Could you check a few things on this model? Use its own coordinates, in mm. Give positions to 0.01 mm unless a question says otherwise; leave off trailing zeros. Order: outer loops, then holes, each group sorted by start corner. A loop starts at its lowest first (then second) coordinate and runs counter-clockwise, first axis right, second up.
from build123d import *

# Parameters (mm, degrees)
SKETCH1_W           = 3
SKETCH1_H           = 6
SKETCH1_W_2         = 6
SKETCH1_H_2         = 3
SKETCH1_W_3         = 50
SKETCH1_H_3         = 50
BOSS_EXTRUDE1_DEPTH = 3
SKETCH2_R           = 2
SKETCH2_W           = 20
SKETCH2_H           = 6.4
CUT_EXTRUDE1_DEPTH  = 76.013332148


with BuildPart() as part:
    # Sketch1 → Boss-Extrude1 (new body)
    with BuildSketch(Plane(origin=(0, 0, 0), x_dir=(1, 0, 0), z_dir=(0, 1, 0))):
        with Locations((-51.5, 9)):
            Rectangle(SKETCH1_W, SKETCH1_H)
        with Locations((-51.5, 25)):
            Rectangle(SKETCH1_W, SKETCH1_H)
        with Locations((-51.5, 41)):
            Rectangle(SKETCH1_W, SKETCH1_H)
        with Locations((-41, 51.5)):
            Rectangle(SKETCH1_W_2, SKETCH1_H_2)
        with Locations((-25, 25)):
            Rectangle(SKETCH1_W_3, SKETCH1_H_3)
        with Locations((-25, 51.5)):
            Rectangle(SKETCH1_W_2, SKETCH1_H_2)
        with Locations((-9, 51.5)):
            Rectangle(SKETCH1_W_2, SKETCH1_H_2)
        with Locations((1.5, 41)):
            Rectangle(SKETCH1_W, SKETCH1_H)
        with Locations((1.5, 25)):
            Rectangle(SKETCH1_W, SKETCH1_H)
        with Locations((1.5, 9)):
            Rectangle(SKETCH1_W, SKETCH1_H)
        with Locations((-9, -1.5)):
            Rectangle(SKETCH1_W_2, SKETCH1_H_2)
        with Locations((-25, -1.5)):
            Rectangle(SKETCH1_W_2, SKETCH1_H_2)
        with Locations((-41, -1.5)):
            Rectangle(SKETCH1_W_2, SKETCH1_H_2)
    extrude(amount=BOSS_EXTRUDE1_DEPTH)

    # Sketch2 → Cut-Extrude1 (cut, through all)
    with BuildSketch(Plane(origin=(0, 3, 0), x_dir=(1, 0, 0), z_dir=(0, 1, 0))):
        with Locations(Location((-40, 10, 0), (0, 0, 270))):
            Circle(SKETCH2_R)
        with Locations(Location((-10, 40, 0), (0, 0, 270))):
            Circle(SKETCH2_R)
        with Locations((-25, 25)):
            Rectangle(SKETCH2_W, SKETCH2_H)
    extrude(amount=-CUT_EXTRUDE1_DEPTH, mode=Mode.SUBTRACT)


solid = part.part
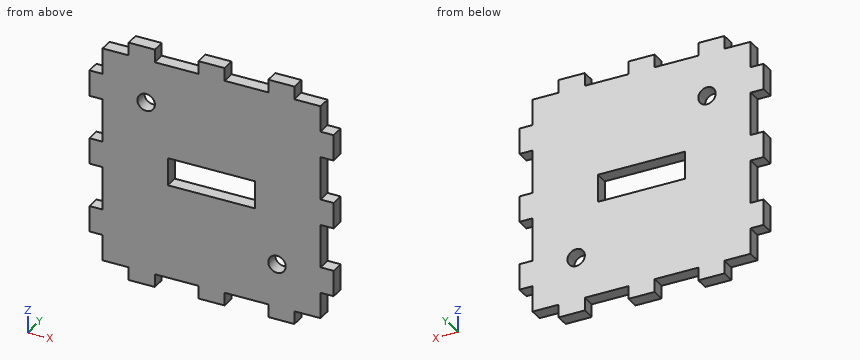
Item 1: Imagine slicing it at D-D on x = -48. List the corners of the cut face in (y, z) for me, then the cut area to 3 significant figures.
Findings:
outline: (0, -50) - (3, -50) - (3, 0) - (0, 0) - close
area: 150 mm2
Item 2: Imagine slicing it at A-A on z = -10. List the corners of the cut face in (x, y) for me, then the cut area to 3 significant figures.
Findings:
outline: (-53, 0) - (-42, 0) - (-42, 3) - (-53, 3) - close; (-38, 0) - (3, 0) - (3, 3) - (-38, 3) - close
area: 156 mm2
Item 3: Imagine slicing it at B-B on x = -40. List the corners of the cut face in (y, z) for me.
Findings:
outline: (0, -53) - (3, -53) - (3, -12) - (0, -12) - close; (0, -8) - (3, -8) - (3, 3) - (0, 3) - close
Item 4: Imagine slicing it at C-C on y = 0.6. Give the number of separate pieces and of enclosed holes in the cut face, then the cut area to 3 significant figures.
Findings:
separate pieces: 1
enclosed holes: 3
area: 2,560 mm2
Item 5: Please list where these lines run through material, in increasing order: line 1 along X through (y, z) = (0.8, -25.5); line 2 along X through (y, z) = (2.35, -10); line 3 along Z through (x, y) = (-27, 2.8).
Findings:
line 1: x = -53 to -35, -15 to 3
line 2: x = -53 to -42, -38 to 3
line 3: z = -53 to -28.2, -21.8 to 3
Item 6: For pin 1 (1.5 mm diameter, centred on x = -51, y = 1, fed in from -Z); pin 2 (6 mm diameter, centred on x = -30.5, z = -6, fed in from -Y); pin 3 (1.5 mm diameter, centred on y = 2, z = -2.5, fed in from -X); pin 4 (0.9 mm diameter, centred on x = -35, y = 2, fed in from +Z), each with a flat end and sliding along its axis, tell me the tip position at first contact or that it passes through.
Findings:
pin 1: stops at z = -44
pin 2: stops at y = 0
pin 3: stops at x = -50
pin 4: stops at z = 0
